Part model, mm, in its own coordinate system. Face numbers are marked on the shaded views. A direction names the side the tool comes from. Coordinates: 2 decimals unless noted, no trailing zeros. Write each loop counter-clockwise with the first axis right and the second up, starting at its lowest first coordinate (ties: lowest second). Pieces come first, ordered by that corner, then holes. Notation, with made-up numbers: M 78,-30 L 135,-30 A27 ccw 135,-7 Z; hole C -39,58 d5. An arc over 180 degrees is marked long. Use a Markdown table: item, result. Add a question column.
Q1. Slice it at C-C on z = 1.25. Write the cut outline in (x, y), then the cut area to 3 significant figures.
Q2. Wall check: L1, parallel to X at y = -1.25, z = 5.25; L2, parallel to Y at x = -1.5, z = 2.25 (3 decimals); L3, parallel to Y at x = -1, z = 3.75. Give the ranges that are in metal, low to high. Write a range as from..to.
Q3. Tool access for the marked faces 5 and 6: list every direction of +Z, -Z, +X, -X, +Y, -Y with a clear straight run to the whole face (end or side of a thin tool).
Q4. Mould opens along Y. For the marked faces 1, 2, 3 and 4 say: released by +Y, released by -Y, zero draft, split by the parting line, or undercut.
Q5. Slice it at A-A on y = 0.75. Write the cut outline in (x, z), then the cut area to 3 significant figures.
Q6. Slice it at D-D on y = -4.25. Write the cut outline in (x, z).
Q7. Slice it at B-B on x = -1.25. Write the cut outline in (y, z).
Q8. Pin check, flat tips, straight feed: pin 1 Ø2 at (x, z) = (0.5, 1.5) entering from +Y; pin 2 Ø2 at (x, z) = (-4, 1.5) entering from +Y. Stop position of each tip, or through.
from build123d import *

# Parameters (mm, degrees)
F1_DEPTH = 7


with BuildPart() as f1:
    # F0 (on Top) → F1 (new body)
    with BuildSketch(Plane.XY):
        Polygon((-5.715768, -3.3), (0, -6.6), (5.715768, -3.3), (5.715768, 3.3), (0, 6.6), (-5.715768, 3.3), align=None)
        with BuildLine():
            ThreePointArc((1.65, 2.137171), (2.423324, 1.190588), (2.7, 0))
            ThreePointArc((2.7, 0), (2.423324, -1.190588), (1.65, -2.137171))
            ThreePointArc((1.65, -2.137171), (0, -2.7), (-1.65, -2.137171))
            ThreePointArc((-1.65, -2.137171), (-2.7, 0), (-1.65, 2.137171))
            ThreePointArc((-1.65, 2.137171), (0, 2.7), (1.65, 2.137171))
        make_face(mode=Mode.SUBTRACT)
        with BuildLine():
            Line((-1.65, -2.137171), (-1.65, 2.137171))
            ThreePointArc((-1.65, 2.137171), (-2.7, 0), (-1.65, -2.137171))
        make_face()
        with BuildLine():
            ThreePointArc((1.65, -2.137171), (2.423324, -1.190588), (2.7, 0))
            ThreePointArc((2.7, 0), (2.423324, 1.190588), (1.65, 2.137171))
            Line((1.65, 2.137171), (1.65, -2.137171))
        make_face()
    extrude(amount=F1_DEPTH)

    # F2 (on Right) → F3 (revolve, cut)
    with BuildSketch(Plane.YZ):
        Polygon((-7.079097, 4.205731), (-5.565229, 8.62103), (-7.079097, 8.62103), align=None)
    revolve(axis=Axis((0, 0, 4.921937), (0, 0, 1)), mode=Mode.SUBTRACT)


solid = f1.part
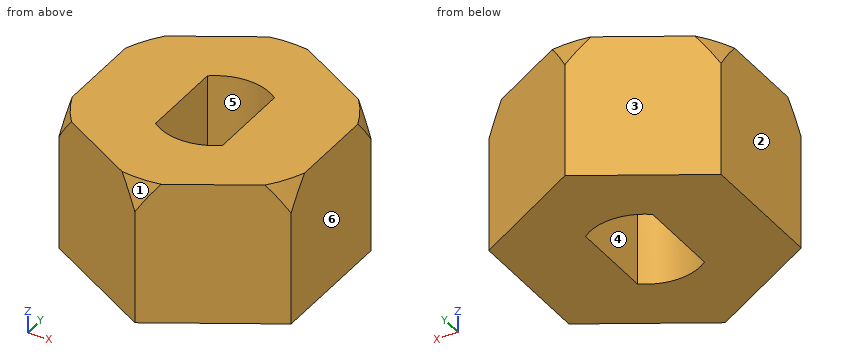
Recorded:
| question | item | result |
|---|---|---|
| 1 | outline | M -5.72,-3.3 L 0,-6.6 L 5.72,-3.3 L 5.72,3.3 L 0,6.6 L -5.72,3.3 Z; hole M -1.65,-2.14 A2.7 ccw 1.65,-2.14 L 1.65,2.14 A2.7 ccw -1.65,2.14 Z |
| 1 | area | 96.5 mm² |
| 2 | L1 | -5.72..-1.65, 1.65..5.72 |
| 2 | L2 | -5.734..-2.245, 2.245..5.734 |
| 2 | L3 | -6.02..-2.51, 2.51..6.02 |
| 3 | face 5 | +Z, -Z |
| 3 | face 6 | +Z, -Z, +X, +Y, -Y |
| 4 | face 1 | released by -Y |
| 4 | face 2 | zero draft |
| 4 | face 3 | released by +Y |
| 4 | face 4 | undercut |
| 5 | outline | M -5.72,0 L -1.65,0 L -1.65,7 L -5.72,7 Z; M 1.65,0 L 5.72,0 L 5.72,7 L 1.65,7 Z |
| 5 | area | 56.9 mm² |
| 6 | outline | M -4.07,0 L 4.07,0 L 4.07,7 L -4.07,7 Z |
| 7 | outline | M -5.88,0 L -2.39,0 L -2.39,7 L -5.88,7 Z; M 2.39,0 L 5.88,0 L 5.88,7 L 2.39,7 Z |
| 8 | pin 1 | y = 6.6 |
| 8 | pin 2 | y = 4.87 |
